For this review, take the finished solid that the model builds, in its own axes (mm). A direction names the side the tool comes from. Give positions to 0.01 mm unless a question says otherwise; leave off trailing zeros. Loops run counter-clockwise (first coordinate to the right, second up) from the corner with the lowest first, then second, coordinate; pieces in that order, holes last.
```python
from build123d import *

# Parameters (mm, degrees)
SKETCH1_R           = 3.25
SKETCH1_R_2         = 1.75
SKETCH1_W           = 7.5
SKETCH1_H           = 7.5
BOSS_EXTRUDE1_DEPTH = 1
SKETCH2_R           = 3.25
SKETCH2_R_2         = 1.75
BOSS_EXTRUDE2_DEPTH = 2.8


with BuildPart() as part:
    # Sketch1 → Boss-Extrude1 (new body)
    # profile 1 of 11: a face of its own
    with BuildSketch(Plane(origin=(0, 0, 0), x_dir=(1, 0, 0), z_dir=(0, 1, 0))):
        with Locations((-15, -15)):
            Circle(SKETCH1_R)
        with Locations(Location((-15, -15, 0), (0, 0, 270))):
            Circle(SKETCH1_R_2, mode=Mode.SUBTRACT)
    # profile 2 of 11: a face of its own
    with BuildSketch(Plane(origin=(0, 0, 0), x_dir=(1, 0, 0), z_dir=(0, 1, 0))):
        with BuildLine():
            add(Edge.make_bspline(
                [(0, -7.5), (-1.930795648, -5.688459272), (-3.75, -3.75)],
                knots=[0.751545437, 0.751545437, 0.751545437, 1, 1, 1], degree=2))
            add(Edge.make_bspline(
                [(-15, -11.75), (-8.240801632, -9.240499337), (-3.75, -3.75)],
                knots=[0, 0, 0, 1, 1, 1], degree=2))
            ThreePointArc((-15, -11.75), (-12.701902961, -12.701902961), (-11.75, -15))
            ThreePointArc((-11.75, -15), (-11.997391519, -16.243721155), (-12.701902961, -17.298097039))
            add(Edge.make_bspline(
                [(-12.701902961, -17.298097039), (-5.840426668, -12.979694751), (0, -7.5)],
                knots=[0, 0, 0, 0.751545437, 0.751545437, 0.751545437], degree=2))
        make_face()
    # profile 3 of 11: a face of its own
    with BuildSketch(Plane(origin=(0, 0, 0), x_dir=(1, 0, 0), z_dir=(0, 1, 0))):
        with BuildLine():
            add(Edge.make_bspline(
                [(0, -7.5), (1.930795648, -5.688459272), (3.75, -3.75)],
                knots=[0.751545437, 0.751545437, 0.751545437, 1, 1, 1], degree=2))
            Line((3.75, -3.75), (-3.75, -3.75))
            add(Edge.make_bspline(
                [(0, -7.5), (-1.930795648, -5.688459272), (-3.75, -3.75)],
                knots=[0.751545437, 0.751545437, 0.751545437, 1, 1, 1], degree=2))
        make_face()
    # profile 4 of 11: a face of its own
    with BuildSketch(Plane(origin=(0, 0, 0), x_dir=(1, 0, 0), z_dir=(0, 1, 0))):
        Rectangle(SKETCH1_W, SKETCH1_H)
    # profile 5 of 11: a face of its own
    with BuildSketch(Plane(origin=(0, 0, 0), x_dir=(1, 0, 0), z_dir=(0, 1, 0))):
        with BuildLine():
            add(Edge.make_bspline(
                [(15, -11.75), (8.240801632, -9.240499337), (3.75, -3.75)],
                knots=[0, 0, 0, 1, 1, 1], degree=2))
            add(Edge.make_bspline(
                [(0, -7.5), (1.930795648, -5.688459272), (3.75, -3.75)],
                knots=[0.751545437, 0.751545437, 0.751545437, 1, 1, 1], degree=2))
            add(Edge.make_bspline(
                [(12.701902961, -17.298097039), (5.840426668, -12.979694751), (0, -7.5)],
                knots=[0, 0, 0, 0.751545437, 0.751545437, 0.751545437], degree=2))
            ThreePointArc((12.701902961, -17.298097039), (11.997391519, -13.756278845), (15, -11.75))
        make_face()
    # profile 6 of 11: a face of its own
    with BuildSketch(Plane(origin=(0, 0, 0), x_dir=(1, 0, 0), z_dir=(0, 1, 0))):
        with Locations((15, -15)):
            Circle(SKETCH1_R)
        with Locations(Location((15, -15, 0), (0, 0, 270))):
            Circle(SKETCH1_R_2, mode=Mode.SUBTRACT)
    # profile 7 of 11: a face of its own
    with BuildSketch(Plane(origin=(0, 0, 0), x_dir=(1, 0, 0), z_dir=(0, 1, 0))):
        with BuildLine():
            add(Edge.make_bspline(
                [(0, 7.5), (1.930795648, 5.688459272), (3.75, 3.75)],
                knots=[0.751545437, 0.751545437, 0.751545437, 1, 1, 1], degree=2))
            add(Edge.make_bspline(
                [(15, 11.75), (8.240801632, 9.240499337), (3.75, 3.75)],
                knots=[0, 0, 0, 1, 1, 1], degree=2))
            ThreePointArc((15, 11.75), (11.997391519, 13.756278845), (12.701902961, 17.298097039))
            add(Edge.make_bspline(
                [(12.701902961, 17.298097039), (5.840426668, 12.979694751), (0, 7.5)],
                knots=[0, 0, 0, 0.751545437, 0.751545437, 0.751545437], degree=2))
        make_face()
    # profile 8 of 11: a face of its own
    with BuildSketch(Plane(origin=(0, 0, 0), x_dir=(1, 0, 0), z_dir=(0, 1, 0))):
        with Locations((15, 15)):
            Circle(SKETCH1_R)
        with Locations(Location((15, 15, 0), (0, 0, 270))):
            Circle(SKETCH1_R_2, mode=Mode.SUBTRACT)
    # profile 9 of 11: a face of its own
    with BuildSketch(Plane(origin=(0, 0, 0), x_dir=(1, 0, 0), z_dir=(0, 1, 0))):
        with BuildLine():
            Line((-3.75, 3.75), (3.75, 3.75))
            add(Edge.make_bspline(
                [(0, 7.5), (1.930795648, 5.688459272), (3.75, 3.75)],
                knots=[0.751545437, 0.751545437, 0.751545437, 1, 1, 1], degree=2))
            add(Edge.make_bspline(
                [(0, 7.5), (-1.930795648, 5.688459272), (-3.75, 3.75)],
                knots=[0.751545437, 0.751545437, 0.751545437, 1, 1, 1], degree=2))
        make_face()
    # profile 10 of 11: a face of its own
    with BuildSketch(Plane(origin=(0, 0, 0), x_dir=(1, 0, 0), z_dir=(0, 1, 0))):
        with BuildLine():
            add(Edge.make_bspline(
                [(-15, 11.75), (-8.240801632, 9.240499337), (-3.75, 3.75)],
                knots=[0, 0, 0, 1, 1, 1], degree=2))
            add(Edge.make_bspline(
                [(0, 7.5), (-1.930795648, 5.688459272), (-3.75, 3.75)],
                knots=[0.751545437, 0.751545437, 0.751545437, 1, 1, 1], degree=2))
            add(Edge.make_bspline(
                [(-12.701902961, 17.298097039), (-5.840426668, 12.979694751), (0, 7.5)],
                knots=[0, 0, 0, 0.751545437, 0.751545437, 0.751545437], degree=2))
            ThreePointArc((-12.701902961, 17.298097039), (-11.997391519, 16.243721155), (-11.75, 15))
            ThreePointArc((-11.75, 15), (-12.701902961, 12.701902961), (-15, 11.75))
        make_face()
    # profile 11 of 11: a face of its own
    with BuildSketch(Plane(origin=(0, 0, 0), x_dir=(1, 0, 0), z_dir=(0, 1, 0))):
        with Locations((-15, 15)):
            Circle(SKETCH1_R)
        with Locations(Location((-15, 15, 0), (0, 0, 270))):
            Circle(SKETCH1_R_2, mode=Mode.SUBTRACT)
    extrude(amount=BOSS_EXTRUDE1_DEPTH)

    # Sketch2 → Boss-Extrude2 (add)
    # profile 1 of 4: a face of its own
    with BuildSketch(Plane(origin=(0, 1, 0), x_dir=(1, 0, 0), z_dir=(0, 1, 0))):
        with Locations(Location((-15, 15, 0), (0, 0, 270))):
            Circle(SKETCH2_R)
        with Locations(Location((-15, 15, 0), (0, 0, 270))):
            Circle(SKETCH2_R_2, mode=Mode.SUBTRACT)
    # profile 2 of 4: a face of its own
    with BuildSketch(Plane(origin=(0, 1, 0), x_dir=(1, 0, 0), z_dir=(0, 1, 0))):
        with Locations(Location((15, 15, 0), (0, 0, 270))):
            Circle(SKETCH2_R)
        with Locations(Location((15, 15, 0), (0, 0, 270))):
            Circle(SKETCH2_R_2, mode=Mode.SUBTRACT)
    # profile 3 of 4: a face of its own
    with BuildSketch(Plane(origin=(0, 1, 0), x_dir=(1, 0, 0), z_dir=(0, 1, 0))):
        with Locations(Location((15, -15, 0), (0, 0, 90))):
            Circle(SKETCH2_R)
        with Locations(Location((15, -15, 0), (0, 0, 270))):
            Circle(SKETCH2_R_2, mode=Mode.SUBTRACT)
    # profile 4 of 4: a face of its own
    with BuildSketch(Plane(origin=(0, 1, 0), x_dir=(1, 0, 0), z_dir=(0, 1, 0))):
        with Locations(Location((-15, -15, 0), (0, 0, 90))):
            Circle(SKETCH2_R)
        with Locations(Location((-15, -15, 0), (0, 0, 270))):
            Circle(SKETCH2_R_2, mode=Mode.SUBTRACT)
    extrude(amount=BOSS_EXTRUDE2_DEPTH)


solid = part.part
```
Item 1: Tool access review of faces 3 (the flat face through (-3.75, 0.5, 0.1)), 4 (the flat face through (16.4, 3.8, 13.6)), 5 (the flat face through (3.75, 0.5, 0.1)), 6 (the flat face through (0, 1, 0)): name each direction out of +Z, -Z, +X, -X, +Y, -Y from which nothing blocks a thin tool from reaching the whole face with its end or side.
Answer:
face 3: -X, +Y, -Y
face 4: +Z, -Z, +X, -X, +Y
face 5: +X, +Y, -Y
face 6: +Y
Item 2: Take a section at B-B on z = 3. Give the boundary of the cut face in (x, y).
Answer:
outline: (-3.75, 0) - (3.75, 0) - (3.75, 1) - (-3.75, 1) - close
Item 3: The part is to be moulded in two halves that separate along Z. For faces 1 (the cylindrical face through (-16.978, 1.873, -17.579)), 2 (the flat face through (13.6, 3.8, -13.6)), say which applies: released by +Z, released by -Z, zero draft, split by the parting line, or undercut.
Answer:
face 1: undercut
face 2: zero draft
Item 4: For L1, parallel to Z at x = 14, y = 2.15; L2, parallel to X at y = 0.55, z = -15; L3, parallel to Z at x = 13.5, y = 0.4, list the stretches that pass through material, from the lowest coordinate up.
Answer:
L1: z = -18.09 to -16.44, -13.56 to -11.91, 11.91 to 13.56, 16.44 to 18.09
L2: x = -18.25 to -16.75, -13.25 to -9.24, 9.24 to 13.25, 16.75 to 18.25
L3: z = -17.88 to -15.9, -14.1 to -11.14, 11.14 to 14.1, 15.9 to 17.88
Item 5: Clearance check with flat-ended pins moving along their axes: pin 1 Ø6 at (x, z) = (5, -8.5) entering from +Y; pin 2 Ø1.1 at (y, z) = (0.5, 0.5) entering from -X. State where each tip first meets the part, or that it passes through.
Answer:
pin 1: stops at y = 1
pin 2: stops at x = -3.75
Item 6: Take a section at C-C on z = -15. State how many separate pieces and enclosed holes the cut face has, and give its area (3 significant figures).
Answer:
separate pieces: 4
enclosed holes: 0
area: 27.8 mm2
Item 7: Take a section at A-A on y = 2.45. Give the boundary of the cut face in (x, z), and give its area (3 significant figures).
Answer:
outline: circle Ø6.5 at (-15, -15); circle Ø6.5 at (-15, 15); circle Ø6.5 at (15, -15); circle Ø6.5 at (15, 15); hole circle Ø3.5 at (-15, -15); hole circle Ø3.5 at (-15, 15); hole circle Ø3.5 at (15, -15); hole circle Ø3.5 at (15, 15)
area: 94.2 mm2
